Model file for the job. Use its own axes, mm. A direction names the side the tool comes from. Coordinates: 2 decimals unless noted, no trailing zeros. Order: outer loops, then holes, each group sorted by start corner. A loop starts at its lowest first (then second) coordinate and runs counter-clockwise, first axis right, second up. Notation, with made-up numbers: (-18, 64) -> (15, 64) arc R26 ccw to (15, 103) -> close; hole circle Ø8 at (71.25, 54). An arc over 180 degrees is marked (long way). Write item = value, one per line. Start each with the question number.
Q1. 3-axis set-ups, long thin cutter, end or side, ignore diameter. For faces 4 (the face through (5, 3.175, 2)), 5 (the face through (-3.175, 5, 3)), 6 (the face through (0, -3.175, 3)): which of +Z, -Z, +X, -X, +Y, -Y reach the whole face in a straight line?
Q2. Cut at C-C, the plane y = 1. List the corners of the cut face in (x, z) (3 decimals), plus the area to 3 significant figures.
Q3. Cut at D-D, the plane x = 6.35. List the corners of the cut face in (y, z) (3 decimals), plus the area to 3 significant figures.
Q4. Cut at B-B, the plane z = 4.25. List the corners of the cut face in (x, y) (1 decimal), plus the area to 3 significant figures.
Q5. Mould opens along Z. For faces 1 (the face through (7.873, -0.044, 3.108)), 2 (the face through (0.192, 6.223, 3.131)), 3 (the face through (0, 1, 0)) say: +Z half, -Z half, draft (parallel to the pull), parting line (faces both ways), or undercut.
Q6. Flat gauge pins, fed straight in: pin 1 (1.1 mm diameter, centred on y = 4.5, z = 3, fed in from +X) (3 decimals); pin 2 (1 mm diameter, centred on y = 5.5, z = 3.5, fed in from -X) (3 decimals). Where does each tip first touch, or does it go through?
Q7. Wall check: line 1 (Y direction, x = 0, z = 5) (1 decimal); line 2 (X direction, y = 0.5, z = 3.25) (3 decimals); line 3 (Z direction, x = -6.35, y = -1.5). Give the ranges that are in metal, low to high. Write a range as from..to.
from build123d import *

# Parameters (mm, degrees)
SKETCH1_W                        = 19.05
SKETCH1_H                        = 6.35
BOSS_EXTRUDE1_DEPTH              = 6.35
SKETCH6_W                        = 6.35
SKETCH6_H                        = 6.35
BOSS_EXTRUDE2_DEPTH              = 4.7625
TAPPED_HOLE_FOR_4_40_HELICOIL1_D = 3.048
F_4_CLEARANCE_HOLE1_D            = 2.9464
DISTINGUISHINGMARK_SIZE          = 1.016


with BuildPart() as part:
    # Sketch1 → Boss-Extrude1 (new body)
    with BuildSketch(Plane.XY):
        Rectangle(SKETCH1_W, SKETCH1_H)
    extrude(amount=BOSS_EXTRUDE1_DEPTH)

    # Sketch6 → Boss-Extrude2 (add)
    with BuildSketch(Plane(origin=(0, 3.175, 0), x_dir=(1, 0, 0), z_dir=(0, 1, 0))):
        with Locations((0, -3.175)):
            Rectangle(SKETCH6_W, SKETCH6_H)
    extrude(amount=BOSS_EXTRUDE2_DEPTH)

    # Tapped Hole for #4-40 Helicoil1 (through all)
    with Locations(Plane(origin=(0, 3.175, 0), x_dir=(1, 0, 0), z_dir=(0, 1, 0))):
        with Locations((-6.35, -3.175), (6.35, -3.175)):
            Hole(TAPPED_HOLE_FOR_4_40_HELICOIL1_D / 2)

    # #4 Clearance Hole1 (through all)
    with Locations(Plane.XY.offset(6.35)):
        with Locations((0, 4.7625)):
            Hole(F_4_CLEARANCE_HOLE1_D / 2)

    # distinguishingMark
    distinguishingmark_edges = [part.edges().sort_by_distance(p)[0] for p in [
        (3.175, 7.9375, 3.175),
        (-3.175, 7.9375, 3.175),
    ]]
    chamfer(distinguishingmark_edges, length=DISTINGUISHINGMARK_SIZE)


solid = part.part
Here are the results:
q1.face_4 = +Z, -Z, +X, +Y
q1.face_5 = +Z, -Z, -X, +Y
q1.face_6 = +Z, -Z, +X, -X, -Y
q2.outline = (-9.525, 0) -> (9.525, 0) -> (9.525, 6.35) -> (-9.525, 6.35) -> close; hole circle Ø3.048 at (-6.35, 3.175); hole circle Ø3.048 at (6.35, 3.175)
q2.area = 106 mm²
q3.outline = (-3.175, 0) -> (3.175, 0) -> (3.175, 1.651) -> (-3.175, 1.651) -> close; (-3.175, 4.699) -> (3.175, 4.699) -> (3.175, 6.35) -> (-3.175, 6.35) -> close
q3.area = 21.0 mm²
q4.outline = (-9.5, -3.2) -> (-7.4, -3.2) -> (-7.4, 3.2) -> (-9.5, 3.2) -> close; (-5.3, -3.2) -> (5.3, -3.2) -> (5.3, 3.2) -> (3.2, 3.2) -> (3.2, 6.9) -> (2.2, 7.9) -> (-2.2, 7.9) -> (-3.2, 6.9) -> (-3.2, 3.2) -> (-5.3, 3.2) -> close; (7.4, -3.2) -> (9.5, -3.2) -> (9.5, 3.2) -> (7.4, 3.2) -> close; hole circle Ø2.9 at (0, 4.8)
q4.area = 116 mm²
q5.face_1 = undercut
q5.face_2 = draft
q5.face_3 = -Z half
q6.pin_1 = 3.175
q6.pin_2 = -3.175
q7.line_1 = -3.2..3.3, 6.2..7.9
q7.line_2 = -9.525..-7.872, -4.828..4.828, 7.872..9.525
q7.line_3 = 0..1.65, 4.7..6.35
